Geometry check sheet. Reference: the model listing, model coordinates, mm. A direction names the side the tool comes from. Coordinates: 2 decimals unless noted, no trailing zeros. Write each loop counter-clockwise with the first axis right and the second up, starting at its lowest first coordinate (ties: lowest second). Pieces come first, ordered by that corner, then holes.
from build123d import *

# Parameters (mm, degrees)
SKETCH1_R           = 7.5
BOSS_EXTRUDE1_DEPTH = 0.5
SKETCH2_R           = 6
BOSS_EXTRUDE2_DEPTH = 15
SKETCH3_R           = 5.5
CUT_EXTRUDE1_DEPTH  = 19.781639971
CHAMFER1_SIZE       = 1


with BuildPart() as part:
    # Sketch1 → Boss-Extrude1 (new body)
    with BuildSketch(Plane.XY):
        Circle(SKETCH1_R)
    extrude(amount=BOSS_EXTRUDE1_DEPTH)

    # Sketch2 → Boss-Extrude2 (add)
    with BuildSketch(Plane(origin=(0, 0, 0), x_dir=(-1, 0, 0), z_dir=(0, 0, -1))):
        Circle(SKETCH2_R)
    extrude(amount=BOSS_EXTRUDE2_DEPTH)

    # Sketch3 → Cut-Extrude1 (cut, through all)
    with BuildSketch(Plane.XY.offset(0.5)):
        Circle(SKETCH3_R)
    extrude(amount=-CUT_EXTRUDE1_DEPTH, mode=Mode.SUBTRACT)

    # Chamfer1
    chamfer1_edges = [part.edges().sort_by_distance(p)[0] for p in [
        (-5.5, 0, 0.5),
        (6, 0, 0),
    ]]
    chamfer(chamfer1_edges, length=CHAMFER1_SIZE)


solid = part.part
1. Sectioned sample at A-A, the plane x = 0. Record the boundary of the cut face in (y, z), and give its area (3 significant figures).
Computed values:
outline: (-7.5, 0) - (-7, 0) - (-6, -1) - (-6, -15) - (-5.5, -15) - (-5.5, -0.5) - (-6.5, 0.5) - (-7.5, 0.5) - close; (5.5, -15) - (6, -15) - (6, -1) - (7, 0) - (7.5, 0) - (7.5, 0.5) - (6.5, 0.5) - (5.5, -0.5) - close
area: 17.0 mm2
2. Thickness scan on line 1 along Y through (x, z) = (0, -8); line 2 along X through (y, z) = (2.5, -9); line 3 along Y through (x, z) = (-0.75, -7.75). Record the ranges inside material, lowest first.
Computed values:
line 1: y = -6 to -5.5, 5.5 to 6
line 2: x = -5.45 to -4.9, 4.9 to 5.45
line 3: y = -5.95 to -5.45, 5.45 to 5.95
3. Sectioned sample at C-C, the plane z = -8.75. Record the boundary of the cut face in (x, y), and give its area (3 significant figures).
Computed values:
outline: circle Ø12 at (0, 0); hole circle Ø11 at (0, 0)
area: 18.1 mm2
4. Sectioned sample at B-B, the plane z = -0.75. Record the boundary of the cut face in (x, y), and give its area (3 significant figures).
Computed values:
outline: circle Ø12.5 at (0, 0); hole circle Ø11 at (0, 0)
area: 27.7 mm2
5. Gauge pin test, flat ends, axial feed: pin 1 Ø5 at (y, z) = (-4.5, -10) entering from +X; pin 2 Ø1.5 at (x, z) = (-2, -9.5) entering from +Y; pin 3 Ø3 at (x, z) = (1, -7.5) entering from +Y. Record the tip position at first contact, or that the pin passes through.
Computed values:
pin 1: stops at x = 5.66
pin 2: stops at y = 5.87
pin 3: stops at y = 6
6. Access from +Z, -Z, +X, -X, +Y, -Y to the whole of each face (thin tool, end or side, straight path). Record for faces 4 (the conical face through (-6, 0, 0)), 5 (the flat face through (7, 2, 0)).
Computed values:
face 4: +Z
face 5: -Z
7. Draft check along X on faces 1 (the flat face through (-3, -5, -15)), 2 (the cylindrical face through (-1.19, -5.37, -7.65)), 3 (the cylindrical face through (6, 0, -8)). Enter one of: released by +X, released by -X, zero draft, split by the parting line, or undercut.
Computed values:
face 1: zero draft
face 2: undercut
face 3: split by the parting line
